CAD build for the part. Positions are in the model's coordinates, mm. Round coordinates to 2 decimals unless told otherwise and drop trailing zeros. Loops run counter-clockwise (first coordinate to the right, second up) from the corner with the lowest first, then second, coordinate; pieces in that order, holes last.
from build123d import *

# Parameters (mm, degrees)
BOSS_EXTRUDE1_DEPTH = 5
SKETCH6_W           = 10
SKETCH6_H           = 15
SKETCH6_R           = 2.5
BOSS_EXTRUDE2_DEPTH = 7


with BuildPart() as part:
    # Sketch5 → Boss-Extrude1 (new, symmetric)
    with BuildSketch(Plane(origin=(0, 0, 0), x_dir=(0, 0, -1), z_dir=(1, 0, 0))):
        with BuildLine():
            Line((-19.663469321, 19.634120506), (-21.416496635, 21.416496635))
            ThreePointArc((-21.416496635, 21.416496635), (9.210493666, 28.853066781), (29.864087216, 5.046677222))
            Line((29.864087216, 5.046677222), (27.321571741, 5.067783672))
            ThreePointArc((27.321571741, 5.067783672), (8.228376229, 26.541374087), (-19.663469321, 19.634120506))
        make_face()
    extrude(amount=BOSS_EXTRUDE1_DEPTH, both=True)

    # Sketch6 → Boss-Extrude2 (add)
    with BuildSketch(Plane(origin=(0, 5.294226257, -0.043949516), x_dir=(1, 0, 0), z_dir=(0, -0.9999655451195217, 0.008301118829285392))):
        with Locations((0, -34.778562105)):
            Rectangle(SKETCH6_W, SKETCH6_H)
        with Locations(Location((0, -36.278562105, 0), (0, 0, 270))):
            Circle(SKETCH6_R, mode=Mode.SUBTRACT)
    extrude(amount=-BOSS_EXTRUDE2_DEPTH)


solid = part.part
Item 1: Cut at B-B (y = 20.25). List the corners of the cut face in (x, z).
Verdict:
outline: (-5, -22.52) - (5, -22.52) - (5, -19.03) - (-5, -19.03) - close; (-5, 19.03) - (5, 19.03) - (5, 20.27) - (-5, 20.27) - close
Item 2: Cut at D-D (z = 4.5). List the corners of the cut face in (x, y).
Verdict:
outline: (-5, 27.42) - (5, 27.42) - (5, 29.95) - (-5, 29.95) - close
Item 3: Mould opens along Z. For faces 1 (the cylindrical face through (0.07, 29.83, -5.25)), 2 (the cylindrical face through (0.07, 26.413, -8.631)), 3 (the flat face through (0.07, 20.513, 20.528)), 4 (the cylindrical face through (-1.521, 8.46, -34.366)) say: released by +Z, released by -Z, zero draft, split by the parting line, or undercut.
Verdict:
face 1: split by the parting line
face 2: undercut
face 3: released by +Z
face 4: undercut
Item 4: Cut at C-C (y = 23.5). List the corners of the cut face in (x, z).
Verdict:
outline: (-5, -19.11) - (5, -19.11) - (5, -14.83) - (-5, -14.83) - close; (-5, 14.83) - (5, 14.83) - (5, 19.11) - (-5, 19.11) - close
Item 5: Flat gauge pins, fed straight in: P1, Ø1, axis at x = 0.5, z = -19.5, coming from the -Y side; P2, Ø2, axis at x = -0.5, y = 11, coming from the +Z side; P3, Ø5, axis at x = 0.5, y = 21.5, coming from the -Z side. Where does each tip first touch, or does it go through?
Verdict:
P1: stops at y = 19.29
P2: stops at z = -25.06
P3: stops at z = -23.59
Item 6: Wall check: L1, parallel to Z at x = 1.25, y = 6.75; L2, parallel to Y at x = 2.75, z = -34.5; L3, parallel to Y at x = -1.5, z = -29. Give the ranges that are in metal, low to high.
Verdict:
L1: z = -42.34 to -38.5, -34.17 to -26.96
L2: y = 5.01 to 12.01
L3: y = 5.05 to 12.05
Item 7: Cut at A-A (x = 1.75). List the corners of the cut face in (y, z) (1 decimal).
Verdict:
outline: (4.9, -42.3) - (11.9, -42.4) - (12, -38.2) - (5, -38.1) - close; (5, -34.5) - (12, -34.6) - (12.1, -27.8) arc R30.3 ccw to (21.4, 21.4) - (19.6, 19.7) arc R27.8 cw to (5.1, -27.3) - close
